Check sheet for the modelled part. Datum: model origin and axes. Units: mm. Face numbers are marked on the shaded views. A direction names the side the tool comes from. Round coordinates to 2 decimals unless told otherwise and drop trailing zeros. Order: outer loops, then holes, each group sorted by start corner. A loop starts at its lowest first (then second) coordinate and runs counter-clockwise, first axis right, second up.
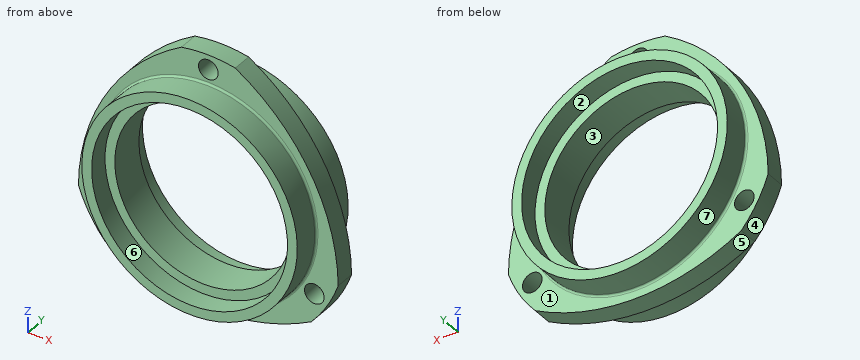
```python
from build123d import *

# Parameters (mm, degrees)
F2_R     = 5
F3_DEPTH = 24.001
F4_R     = 81.962232
F5_DEPTH = 24.001
F6_R     = 1


with BuildPart() as f1:
    # F0 (on Right) → F1 (revolve)
    with BuildSketch(Plane.YZ):
        Polygon((-19, 55), (-19, 50), (-9, 50), (-9, 45), (9, 45), (9, 50), (19, 50), (19, 55), (5, 55), (5, 70), (-5, 70), (-5, 55), align=None)
    revolve(axis=Axis((0, 0.467166, 0), (0, 1, 0)))

    # F2 (on face) → F3 (cut, through all)
    with BuildSketch(Plane.XZ.offset(5)):
        with Locations((0, 62.5)):
            Circle(F2_R)
        with Locations((-54.126588, -31.25)):
            Circle(F2_R)
        with Locations((54.126588, -31.25)):
            Circle(F2_R)
    extrude(amount=-F3_DEPTH, mode=Mode.SUBTRACT)

    # F4 (on face) → F5 (cut, through all)
    with BuildSketch(Plane.XZ.offset(5)):
        Circle(F4_R)
        with BuildLine():
            ThreePointArc((-13.741895, 68.637893), (0, 70), (13.741895, 68.637893))
            ThreePointArc((13.741895, 68.637893), (51.961524, 30), (66.313106, -22.418116))
            ThreePointArc((66.313106, -22.418116), (60.621778, -35), (52.571211, -46.219777))
            ThreePointArc((52.571211, -46.219777), (0, -60), (-52.571211, -46.219777))
            ThreePointArc((-52.571211, -46.219777), (-60.621778, -35), (-66.313106, -22.418116))
            ThreePointArc((-66.313106, -22.418116), (-51.961524, 30), (-13.741895, 68.637893))
        make_face(mode=Mode.SUBTRACT)
    extrude(amount=-F5_DEPTH, mode=Mode.SUBTRACT)

    # F6
    f6_edges = [f1.edges().sort_by_distance(p)[0] for p in [
        (0, -5, -55),
        (0, 5, -55),
    ]]
    fillet(f6_edges, radius=F6_R)


solid = f1.part
```
Item 1: Go/stop test with flat-tipped pins: P1, Ø2, axis at y = -4, z = 0, coming from the -X side; P2, Ø3, axis at x = 45.5, z = -13.5, coming from the -Y side; P3, Ø16, axis at x = -54.13, z = -31.25, coming from the +Y side; P4, Ø3, axis at x = 6.5, z = 45.5, coming from the +Y side. Record where each tip stops, or that it passes through.
Answer:
P1: stops at x = -63.91
P2: stops at y = -9
P3: stops at y = 19
P4: stops at y = 9
Item 2: Sectioned sample at D-D (z = 0). Record the cut outline in (x, y), and give its area (3 significant figures).
Answer:
outline: (-63.69, -5) - (-56, -5) arc R1 cw to (-55, -6) - (-55, -19) - (-50, -19) - (-50, -9) - (-45, -9) - (-45, 9) - (-50, 9) - (-50, 19) - (-55, 19) - (-55, 6) arc R1 cw to (-56, 5) - (-63.69, 5) - close; (45, -9) - (50, -9) - (50, -19) - (55, -19) - (55, -6) arc R1 cw to (56, -5) - (63.69, -5) - (63.69, 5) - (56, 5) arc R1 cw to (55, 6) - (55, 19) - (50, 19) - (50, 9) - (45, 9) - close
area: 735 mm2
Item 3: Sectioned sample at A-A (y = 1). Record the cut outline in (x, z), and give its area (3 significant figures).
Answer:
outline: (-66.31, -22.42) arc R70 ccw to (-52.57, -46.22) arc R107.17 ccw to (52.57, -46.22) arc R70 ccw to (66.31, -22.42) arc R107.17 ccw to (13.74, 68.64) arc R70 ccw to (-13.74, 68.64) arc R107.17 ccw to start; hole circle Ø10 at (-54.13, -31.25); hole circle Ø90 at (0, 0); hole circle Ø10 at (0, 62.5); hole circle Ø10 at (54.13, -31.25)
area: 6,530 mm2
Item 4: Release check for a two-part mould opening along Z. For the marked faces 1, 2, 3 and 4 record: released by +Z, released by -Z, zero draft, split by the parting line, or undercut.
Answer:
face 1: zero draft
face 2: undercut
face 3: undercut
face 4: released by -Z
Item 5: Access from +Z, -Z, +X, -X, +Y, -Y to the whole of each face (thin tool, end or side, straight path). Record for the marked faces 5, 6 and 7.
Answer:
face 5: -Z, +Y, -Y
face 6: -Y
face 7: +Y
Item 6: Scan lines: line 1 along X through (y, z) = (14.5, 0); line 2 along Y through (x, z) = (-30, -54); line 3 along Z through (x, y) = (-14.5, -11.5). Record each from-to range of solid material in increasing order.
Answer:
line 1: x = -55 to -50, 50 to 55
line 2: y = -5 to 5
line 3: z = -53.05 to -47.85, 47.85 to 53.05
Item 7: Sectioned sample at C-C (z = 62.5). Record the cut outline in (x, y), and give its area (3 significant figures).
Answer:
outline: (-22.98, -5) - (-5, -5) - (-5, 5) - (-22.98, 5) - close; (5, -5) - (22.98, -5) - (22.98, 5) - (5, 5) - close
area: 360 mm2
Item 8: Sectioned sample at B-B (x = 0). State how many separate pieces and enclosed holes the cut face has, and give its area (3 significant figures).
Answer:
separate pieces: 3
enclosed holes: 0
area: 661 mm2
